Design review of the part built by this model. Coordinates are the model's own, in mm. A direction names the side the tool comes from. Coordinates: 2 decimals unless noted, no trailing zeros. Loops run counter-clockwise (first coordinate to the right, second up) from the corner with the lowest first, then second, coordinate; pieces in that order, holes last. Notation, with made-up numbers: M 64,-39.75 L 86,-39.75 A26 ccw 86,-3.75 Z; hole C 69.25,14 d2. An arc over 180 degrees is marked long. Answer as a JSON object with one key per item and string values. Group by question number.
1. Insertion check: pin 1 (6 mm diameter, centred on x = -55, z = -33.5, fed in from -Y); pin 2 (12.5 mm diameter, centred on y = 258.32, z = -37.68, fed in from -X). Each pin has a flat end and moves straight along its axis. Give the tip position at first contact, or say it passes through.
2. To check wall thickness, follow probe 1 along Z at (x, y) = (-36.75, 329); probe 2 along X at (y, z) = (701, -41.25); probe 3 along Y at (x, z) = (-35, -32) (3 decimals). State the ranges of each line that lie inside material, in increasing order.
3. Draft analysis for pull direction Y (two halves, no side actions). For faces 1 (the flat face through (-47, 459, -50.377)), 2 (the cylindrical face through (-34.706, 258.667, -29.747)), 3 (the flat face through (-35.307, 61.103, -37.736)), state which applies: +Y half, -Y half, draft (parallel to the pull), parting line (faces both ways), or undercut.
4. Consider section C-C (z = -37). State the section outline as (x, y) points.
5. Consider section A-A (x = -52). State the section outline as (y, z) points.
6. Consider section B-B (y = 212). State the section outline as (x, z) points, then the cut area to 3 significant figures.
7. Machinability: for faces 4 (the flat face through (-48.477, 863.972, -49.285)), 5 (the flat face through (-33.955, 465, -37)), 6 (the flat face through (-47, 458, -48.853)), which of the approach directions +Z, -Z, +X, -X, +Y, -Y give a long, thin tool a straight path to every point of the face, cutting with its end or side? Answer none if there is none.
from build123d import *

# Parameters (mm, degrees)
SKETCH1_W               = 25.4
SKETCH1_H               = 25.4
SKETCH1_W_2             = 22.352
SKETCH1_H_2             = 22.352
BOSS_EXTRUDE1_DEPTH     = 883.666
SKETCH5_R               = 7.9375
CUT_EXTRUDE3_DEPTH      = 1
CUT_EXTRUDE3_DEPTH_BACK = 26.4
SKETCH6_R               = 7.9375
CUT_EXTRUDE4_DEPTH      = 1
CUT_EXTRUDE4_DEPTH_BACK = 26.4
CUT_EXTRUDE5_DEPTH      = 1
CUT_EXTRUDE5_DEPTH_BACK = 26.4
CUT_EXTRUDE6_DEPTH      = 1
CUT_EXTRUDE6_DEPTH_BACK = 26.4


with BuildPart() as part:
    # Sketch1 → Boss-Extrude1 (new body)
    with BuildSketch(Plane(origin=(0, 0, 0), x_dir=(1, 0, 0), z_dir=(0, 1, 0))):
        with Locations((-46.655111286, 37.676591231)):
            Rectangle(SKETCH1_W, SKETCH1_H)
        with Locations((-46.655111286, 37.676591231)):
            Rectangle(SKETCH1_W_2, SKETCH1_H_2, mode=Mode.SUBTRACT)
    extrude(amount=BOSS_EXTRUDE1_DEPTH)

    # Sketch5 → Cut-Extrude3 (cut, two sides)
    with BuildSketch(Plane(origin=(-33.955111286, 0, 0), x_dir=(0, 0, -1), z_dir=(1, 0, 0))) as cut_extrude3_sk:
        with Locations((37.676591231, 258.318)):
            Circle(SKETCH5_R)
    extrude(amount=CUT_EXTRUDE3_DEPTH, mode=Mode.SUBTRACT)
    extrude(cut_extrude3_sk.sketch, amount=-CUT_EXTRUDE3_DEPTH_BACK, mode=Mode.SUBTRACT)

    # Sketch6 → Cut-Extrude4 (cut, two sides)
    with BuildSketch(Plane(origin=(-33.955111286, 0, 0), x_dir=(0, 0, -1), z_dir=(1, 0, 0))) as cut_extrude4_sk:
        with Locations((37.676591231, 813.943)):
            Circle(SKETCH6_R)
    extrude(amount=CUT_EXTRUDE4_DEPTH, mode=Mode.SUBTRACT)
    extrude(cut_extrude4_sk.sketch, amount=-CUT_EXTRUDE4_DEPTH_BACK, mode=Mode.SUBTRACT)

    # Sketch7 → Cut-Extrude5 (cut, two sides)
    with BuildSketch(Plane(origin=(-33.955111286, 0, 0), x_dir=(0, 0, -1), z_dir=(1, 0, 0))) as cut_extrude5_sk:
        Polygon((24.976591231, 883.666), (31.52840716, 859.214290072), (50.376591231, 864.264645773), (50.376591231, 883.666), align=None)
    extrude(amount=CUT_EXTRUDE5_DEPTH, mode=Mode.SUBTRACT)
    extrude(cut_extrude5_sk.sketch, amount=-CUT_EXTRUDE5_DEPTH_BACK, mode=Mode.SUBTRACT)

    # Sketch8 → Cut-Extrude6 (cut, two sides)
    with BuildSketch(Plane(origin=(-33.955111286, 0, 0), x_dir=(0, 0, -1), z_dir=(1, 0, 0))) as cut_extrude6_sk:
        Polygon((24.976591231, 57.658), (24.976591231, 0), (50.376591231, 0), (50.376591231, 64.516), align=None)
    extrude(amount=CUT_EXTRUDE6_DEPTH, mode=Mode.SUBTRACT)
    extrude(cut_extrude6_sk.sketch, amount=-CUT_EXTRUDE6_DEPTH_BACK, mode=Mode.SUBTRACT)


solid = part.part
Findings below:
{
 "1": {"pin 1": "stops at y = 59.69", "pin 2": "passes through"},
 "2": {"probe 1": "z = -50.38 to -48.85, -26.5 to -24.98", "probe 2": "x = -59.36 to -57.83, -35.48 to -33.96", "probe 3": "y = 59.554 to 252.77, 263.866 to 808.395, 819.491 to 859.341"},
 "3": {"face 1": "draft", "face 2": "undercut", "face 3": "-Y half"},
 "4": {"outline": "M -59.36,60.9 L -57.83,60.9 L -57.83,250.41 L -59.36,250.41 Z; M -59.36,266.23 L -57.83,266.23 L -57.83,806.03 L -59.36,806.03 Z; M -59.36,821.85 L -57.83,821.85 L -57.83,860.68 L -59.36,860.68 Z; M -35.48,60.9 L -33.96,60.9 L -33.96,250.41 L -35.48,250.41 Z; M -35.48,266.23 L -33.96,266.23 L -33.96,806.03 L -35.48,806.03 Z; M -35.48,821.85 L -33.96,821.85 L -33.96,860.68 L -35.48,860.68 Z"},
 "5": {"outline": "M 57.66,-24.98 L 58.07,-26.5 L 877.98,-26.5 L 883.67,-24.98 Z; M 64.1,-48.85 L 64.52,-50.38 L 864.26,-50.38 L 863.86,-48.85 Z"},
 "6": {"outline": "M -59.36,-50.38 L -33.96,-50.38 L -33.96,-24.98 L -59.36,-24.98 Z; hole M -57.83,-48.85 L -35.48,-48.85 L -35.48,-26.5 L -57.83,-26.5 Z", "area": "146 mm^2"},
 "7": {"face 4": "+X, -X, +Y", "face 5": "+Z, -Z, +X, +Y, -Y", "face 6": "+Y, -Y"}
}
